Work out the finished part from the listing and answer in its coordinate system (mm). A direction names the side the tool comes from. Round coordinates to 2 decimals unless told otherwise and drop trailing zeros. Write each loop counter-clockwise with the first axis right and the second up, starting at its lowest first coordinate (ties: lowest second). Pieces come first, ordered by that corner, then holes. Notation, with made-up numbers: M -13.5,83.5 L 19.5,83.5 A23 ccw 19.5,93.5 Z; hole C 6,12 d7. An arc over 180 degrees is marked long. Answer in a Markdown table with one row per item.
```python
from build123d import *

# Parameters (mm, degrees)
SKETCH_1_W          = 20
SKETCH_1_H          = 20
SKETCH_1_W_2        = 16
SKETCH_1_H_2        = 16
EXTRUDE_1_DEPTH     = 560
SKETCH_3_R          = 2.2
CUT_EXTRUDE_2_DEPTH = 560
SKETCH_4_R          = 2.2
CUT_EXTRUDE_3_DEPTH = 560
SKETCH_5_W          = 35.553041162
SKETCH_5_H          = 54.410354854
CUT_EXTRUDE_4_DEPTH = 40
SKETCH_6_W          = 32.938502486
SKETCH_6_H          = 36.721798984
CUT_EXTRUDE_5_DEPTH = 40
SKETCH_8_R          = 1
CUT_EXTRUDE_7_DEPTH = 10
SKETCH_10_R         = 2.1
CUT_EXTRUDE_8_DEPTH = 21
SKETCH_11_R         = 6
CUT_EXTRUDE_9_DEPTH = 10
M4X0_7_1_D          = 3.3
M4X0_7_1_DEPTH      = 11.5
M4X0_7_1_TIP        = 0.991420021


with BuildPart() as part:
    # ｽｹｯﾁ1 → ﾎﾞｽ - 押し出し1 (new body)
    with BuildSketch(Plane.XY):
        Rectangle(SKETCH_1_W, SKETCH_1_H)
        Rectangle(SKETCH_1_W_2, SKETCH_1_H_2, mode=Mode.SUBTRACT)
    extrude(amount=EXTRUDE_1_DEPTH)

    # ｽｹｯﾁ3 → ｶｯﾄ - 押し出し2 (cut)
    with BuildSketch(Plane(origin=(10, 0, 0), x_dir=(0, 0, -1), z_dir=(1, 0, 0))):
        with Locations((-530, 0)):
            Circle(SKETCH_3_R)
        with Locations((-30, 0)):
            Circle(SKETCH_3_R)
    extrude(amount=-CUT_EXTRUDE_2_DEPTH, mode=Mode.SUBTRACT)

    # ｽｹｯﾁ4 → ｶｯﾄ - 押し出し3 (cut)
    with BuildSketch(Plane(origin=(0, 10, 0), x_dir=(1, 0, 0), z_dir=(0, 1, 0))):
        with Locations((0, -550)):
            Circle(SKETCH_4_R)
        with Locations((0, -10)):
            Circle(SKETCH_4_R)
    extrude(amount=-CUT_EXTRUDE_3_DEPTH, mode=Mode.SUBTRACT)

    # ｽｹｯﾁ5 → ｶｯﾄ - 押し出し4 (cut)
    with BuildSketch(Plane(origin=(0, 0, 0), x_dir=(-1, 0, 0), z_dir=(0, 0, -1))):
        Rectangle(SKETCH_5_W, SKETCH_5_H)
    extrude(amount=-CUT_EXTRUDE_4_DEPTH, mode=Mode.SUBTRACT)

    # ｽｹｯﾁ6 → ｶｯﾄ - 押し出し5 (cut)
    with BuildSketch(Plane.XY.offset(560)):
        Rectangle(SKETCH_6_W, SKETCH_6_H)
    extrude(amount=-CUT_EXTRUDE_5_DEPTH, mode=Mode.SUBTRACT)

    # ｽｹｯﾁ8 → ｶｯﾄ - 押し出し7 (cut)
    with BuildSketch(Plane(origin=(10, 0, 0), x_dir=(0, 0, -1), z_dir=(1, 0, 0))):
        with Locations((-50, 0)):
            Circle(SKETCH_8_R)
        with Locations((-70, 0)):
            Circle(SKETCH_8_R)
        with Locations((-490, 0)):
            Circle(SKETCH_8_R)
        with Locations((-510, 0)):
            Circle(SKETCH_8_R)
    extrude(amount=-CUT_EXTRUDE_7_DEPTH, mode=Mode.SUBTRACT)

    # ｽｹｯﾁ10 → ｶｯﾄ - 押し出し8 (cut, through all)
    with BuildSketch(Plane.XZ.offset(10)):
        with Locations((0, 234)):
            Circle(SKETCH_10_R)
    extrude(amount=-CUT_EXTRUDE_8_DEPTH, mode=Mode.SUBTRACT)

    # ｽｹｯﾁ11 → ｶｯﾄ - 押し出し9 (cut)
    with BuildSketch(Plane.XZ.offset(10)):
        with Locations((0, 234)):
            Circle(SKETCH_11_R)
    extrude(amount=-CUT_EXTRUDE_9_DEPTH, mode=Mode.SUBTRACT)

    # M4x0.7 ねじ穴1
    with Locations(Plane(origin=(10, 0, 50), x_dir=(0, 0, 1), z_dir=(1, 0, 0))):
        with Locations((0, 0), (20, 0), (440, 0), (460, 0)):
            Hole(M4X0_7_1_D / 2, depth=M4X0_7_1_DEPTH)
            with Locations((0, 0, -(M4X0_7_1_DEPTH + M4X0_7_1_TIP / 2))):  # 118° drill point
                Cone(0, M4X0_7_1_D / 2, M4X0_7_1_TIP, mode=Mode.SUBTRACT)


solid = part.part
```
1. Given pin 1 (2.5 mm diameter, centred on y = 0, z = 50, fed in from +X); pin 2 (11 mm diameter, centred on x = 0, z = 234, fed in from -Y), each flat-ended and moving along its own axis, determine where each tip first touches the part or whether it passes through.
Calculated:
| item | result |
|---|---|
| pin 1 | stops at x = -8 |
| pin 2 | stops at y = 8 |
2. Determine the mould class of faces 3 (the cylindrical face through (-0.78, -9.01, 239.95)), 4 (the flat face through (-10, 0, 277)), 5 (the flat face through (0, -10, 277)) for opening direction X: released by +X, released by -X, zero draft, split by the parting line, or undercut.
Calculated:
| item | result |
|---|---|
| face 3 | undercut |
| face 4 | released by -X |
| face 5 | zero draft |
3. Consider line 1 along Y through (x, z) = (9.1, 70); line 2 along X through (y, z) = (-4, 196.5). Determine where each line is inside the solid, lowest interval first. Write a range as from..to.
Calculated:
| item | result |
|---|---|
| line 1 | y = -10..-1.65, 1.65..10 |
| line 2 | x = -10..-8, 8..10 |
4. The part is cut by section A-A (z = 425.5). Determine the outline of the cut face in (x, y), plus the area to 3 significant figures.
Calculated:
| item | result |
|---|---|
| outline | M -10,-10 L 10,-10 L 10,10 L -10,10 Z; hole M -8,-8 L 8,-8 L 8,8 L -8,8 Z |
| area | 144 mm² |
5. A tool of negligible diameter and unlimited length cuts with its end or side. For faces 1 (the flat face through (10, 0, 277)), 2 (the flat face through (0, -8, 277)), from which of +Z, -Z, +X, -X, +Y, -Y can it reach the whole face along a straight path? Write none if from no direction.
Calculated:
| item | result |
|---|---|
| face 1 | +Z, -Z, +X, +Y, -Y |
| face 2 | +Z, -Z |
